Part model, mm, in its own coordinate system. Coordinates: 2 decimals unless noted, no trailing zeros. Order: outer loops, then holes, each group sorted by start corner. A loop starts at its lowest first (then second) coordinate and runs counter-clockwise, first axis right, second up.
from build123d import *

# Parameters (mm, degrees)
CROQUIS1_W              = 48
CROQUIS1_H              = 6
SALIENTE_EXTRUIR1_DEPTH = 80
CROQUIS6_R              = 2
CORTAR_EXTRUIR4_DEPTH   = 84.737685662


with BuildPart() as part:
    # Croquis1 → Saliente-Extruir1 (new body)
    with BuildSketch(Plane.XY):
        Rectangle(CROQUIS1_W, CROQUIS1_H)
    extrude(amount=SALIENTE_EXTRUIR1_DEPTH)

    # Croquis6 → Cortar-Extruir4 (cut, through all)
    with BuildSketch(Plane.XZ.offset(3)):
        with Locations(Location((16, 61.2, 0), (0, 0, 270))):
            Circle(CROQUIS6_R)
        with Locations(Location((18, 36.8, 0), (0, 0, 270))):
            Circle(CROQUIS6_R)
        with Locations(Location((18, 18.8, 0), (0, 0, 270))):
            Circle(CROQUIS6_R)
        with Locations(Location((-17, 61.2, 0), (0, 0, 270))):
            Circle(CROQUIS6_R)
        with Locations(Location((-15, 36.8, 0), (0, 0, 270))):
            Circle(CROQUIS6_R)
        with Locations(Location((-15, 18.8, 0), (0, 0, 270))):
            Circle(CROQUIS6_R)
        with Locations(Location((-17, 43.2, 0), (0, 0, 270))):
            Circle(CROQUIS6_R)
        with Locations(Location((16, 43.2, 0), (0, 0, 270))):
            Circle(CROQUIS6_R)
    extrude(amount=-CORTAR_EXTRUIR4_DEPTH, mode=Mode.SUBTRACT)


solid = part.part
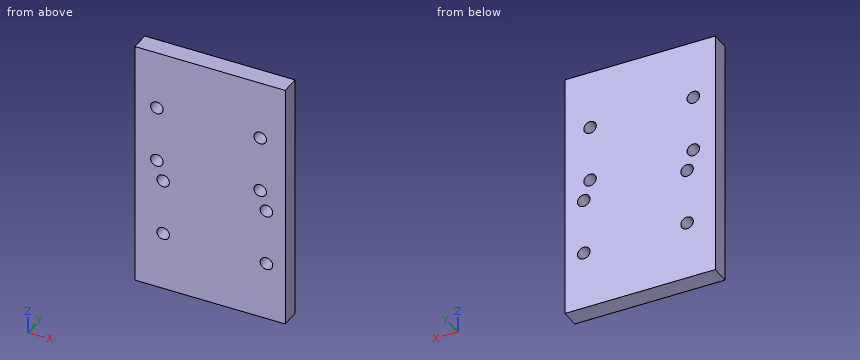
Q1. Cut at B-B on y = 0.9. Count the separate pieces of the cut face and the enclosed holes in it, and give its area (3 significant figures).
Results list:
separate pieces: 1
enclosed holes: 8
area: 3,740 mm2
Q2. Cut at A-A on z = 61.2. Write the cut outline in (x, y).
Results list:
outline: (-24, -3) - (-19, -3) - (-19, 3) - (-24, 3) - close; (-15, -3) - (14, -3) - (14, 3) - (-15, 3) - close; (18, -3) - (24, -3) - (24, 3) - (18, 3) - close
Q3. Pin check, flat tip, straight feed: pin 1 Ø3.5 at (x, z) = (-15, 18.8) entering from +Y. Stop position of the tip, or through.
Results list:
pin 1: passes through
Q4. Wall check: line 1 along X through (y, z) = (-0.05, 36.8); line 2 along X through (y, z) = (-0.25, 61.2); line 3 along Z through (x, y) = (-16.5, -2.25). Give the ranges that are in metal, low to high.
Results list:
line 1: x = -24 to -17, -13 to 16, 20 to 24
line 2: x = -24 to -19, -15 to 14, 18 to 24
line 3: z = 0 to 17.48, 20.12 to 35.48, 38.12 to 41.26, 45.14 to 59.26, 63.14 to 80
Q5. Cut at C-C on z = 43. Write the cut outline in (x, y).
Results list:
outline: (-24, -3) - (-18.99, -3) - (-18.99, 3) - (-24, 3) - close; (-15.01, -3) - (14.01, -3) - (14.01, 3) - (-15.01, 3) - close; (17.99, -3) - (24, -3) - (24, 3) - (17.99, 3) - close
